Autodesk Inventor part; units mm, degrees
ref_plane "Work Plane1" through (0, 0, -5) normal (0, 0, 1) x (1, 0, 0)
ref_plane "YZ Plane" through (0, 0, 0) normal (1, 0, 0) x (0, 1, 0)
ref_plane "XZ Plane" through (0, 0, 0) normal (0, 1, 0) x (-1, 0, 0)
sketch "Sketch1" plane through (0, 0, 0) normal (0, 1, 0) x (-1, 0, 0)
  circle A0 centre (0, 0) radius 5
  dimension "d0" = 10
extrude "Extrusion1" add sketch "Sketch1" along normal blind 32
sketch "Sketch2" plane through (0, 32, 0) normal (0, 1, 0) x (1, 0, 0)
  line L0 (-1.5, 5) -> (1.5, 5)
  line L1 (1.5, 5) -> (1.5, -5)
  line L2 (1.5, -5) -> (-1.5, -5)
  line L3 (-1.5, -5) -> (-1.5, 5)
  point P0 (0, 0)
  point P1 (-1.5, 0)
  point P2 (0, 5)
  dimension "d3" = 3
  dimension "d4" = 10
extrude "Extrusion2" cut sketch "Sketch2" against normal blind 8
sketch "Sketch3" plane through (1.5, 32, -4.7697) normal (-1, 0, 0) x (0, 0, 1)
  circle A0 centre (4.7697, -3) radius 1
  line L0 (9.5394, 0) -> (0, 0)
  point P0 (4.7697, -32)
  point P1 (4.7697, 0)
  dimension "d7" = 2
  dimension "d8" = 3
extrude "Extrusion3" add sketch "Sketch3" along normal blind 3
ref_plane "Work Plane1" through (0, 0, -5) normal (0, 0, 1) x (1, 0, 0)
sketch "Sketch5" plane through (0, 0, -5) normal (0, 0, 1) x (1, 0, 0)
  point P0 (0, 0)
  point P1 (0, 7)
  dimension "d14" = 7
hole "Hole1" at (0, 7, -5) direction (0, 0, 1) diameter 3.302 end through all countersink diameter 8 countersink angle 90
equation "\"d20\" = Thickness"
equation "\"BendRadius\" = Thickness"
equation "\"BendReliefWidth\" = Thickness"
equation "\"BendReliefDepth\" = 0.5 * Thickness"
equation "\"CornerReliefSize\" = 4 * Thickness"
equation "\"MinimumRemnant\" = 2 * Thickness"
equation "\"TransitionRadius\" = BendRadius"
equation "\"JacobiRadiusSize\" = BendRadius"
equation "\"GapSize\" = Thickness"
properties part number "barrel_hinge-female" material "Stainless Steel"
The model under review builds one solid part; all positions refer to its coordinate system, in mm. A direction names the side the tool comes from. Round coordinates to 2 decimals unless told otherwise and drop trailing zeros. Write each loop counter-clockwise with the first axis right and the second up, starting at its lowest first coordinate (ties: lowest second). Pieces come first, ordered by that corner, then holes.
(1) Machinability: for faces 5 (the cylindrical face through (0, 28, 0)), 6 (the flat face through (-3, 32, 0)), which of the approach directions +Z, -Z, +X, -X, +Y, -Y give a long, thin tool a straight path to every point of the face, cutting with its end or side? Answer none if there is none.
(2) We need section A-A on x = 0. Give the boundary of the cut face in (y, z), and give its area (3 significant figures).
(3) We need section D-D on z = -3.25. Give the boundary of the cut face in (x, y).
(4) Insertion check: pin 1 (6 mm diameter, centred on y = 21, z = 3.5, fed in from +X); pin 2 (0.9 mm diameter, centred on x = -0.5, z = -1, fed in from +Y); pin 3 (4 mm diameter, centred on x = 3.5, y = 3, fed in from -Z). Each pin has a flat end and moves straight along its axis. Give the tip position at first contact, or say it passes through.
(5) We need section B-B on z = 0. Give the boundary of the cut face in (x, y).
(6) We need section C-C on y = 29. Give the boundary of the cut face in (x, z).
(7) Mouldability with a two-part tool opening along X and no side actions: class faces 1 (the flat face through (1.5, 27, 0)), 2 (the cylindrical face through (-2.307, 15.776, 4.436)), 3 (the conical face through (0, 5, -3)), 4 (the flat face through (0, 0, 0)) as +X half, -X half, draft (parallel to the pull), parting line (faces both ways), or undercut.
(8) Wall thickness on L1, parallel to Y at x = 0, z = 1.5; L2, parallel to X at y = 7, z = 1.5; L3, parallel to Y at x = -0.5, z = 0: over which ranges is each line inside the solid? List them lowest first.
Findings below:
1. face 5: none
1. face 6: +Z, -Z, +X, -X, +Y
2. outline: (0, -5) - (3, -5) - (5.35, -2.65) - (5.35, 5) - (0, 5) - close; (8.65, -2.65) - (11, -5) - (24, -5) - (24, 5) - (8.65, 5) - close; circle Ø2 at (29, 0)
2. area: 205 mm2
3. outline: (-3.8, 0) - (3.8, 0) - (3.8, 32) - (1.5, 32) - (1.5, 24) - (-1.5, 24) - (-1.5, 32) - (-3.8, 32) - close; hole circle Ø4.5 at (0, 7)
4. pin 1: stops at x = 4.97
4. pin 2: stops at y = 29.84
4. pin 3: stops at z = -4.77
5. outline: (-5, 0) - (5, 0) - (5, 32) - (1.5, 32) - (1.5, 30) - (-1.5, 30) - (-1.5, 32) - (-5, 32) - close; hole circle Ø3.3 at (0, 7); hole (-1.5, 24) - (1.5, 24) - (1.5, 28) - (-1.5, 28) - close
6. outline: (-1.5, -4.77) - (-1.5, -1) - (1.5, -1) - (1.5, -4.77) arc R5 ccw to (1.5, 4.77) - (1.5, 1) - (-1.5, 1) - (-1.5, 4.77) arc R5 ccw to start
7. face 1: undercut
7. face 2: parting line
7. face 3: undercut
7. face 4: draft
8. L1: y = 0 to 5.35, 8.65 to 24
8. L2: x = -4.77 to -1.65, 1.65 to 4.77
8. L3: y = 0 to 5.43, 8.57 to 24, 28 to 30
